CAD build for the part. Positions are in the model's coordinates, mm. A direction names the side the tool comes from. Coordinates: 2 decimals unless noted, no trailing zeros. Write each loop counter-clockwise with the first axis right and the second up, starting at its lowest first coordinate (ties: lowest second). Pieces come first, ordered by that corner, then holes. Notation, with made-up numbers: (15.5, 46) - (57.5, 46) arc R30 cw to (57.5, 80) - close; hole circle Ø8 at (10.5, 72). An arc over 180 degrees is marked (long way). One line per question, with ' | ' between items. Start each with the question number.
1. Which spindle directions (+Z, -Z, +X, -X, +Y, -Y) get a long thin tool onto all of the face, cutting with end or side? Do faces 1 (the cylindrical face through (66.182, 20.26, 100.327)), 2 (the flat face through (114.63, 10.353, 118.958)), 3 (the flat face through (103, 11, 0)). Say none if no direction does.
2. Band-saw the part on A-A, the plane x = 97. Write the cut outline in (y, z), then the cut area to 3 significant figures.
3. Two-plate mould, pull along X, no slides. Class faces 4 (the flat face through (0, 11, 92)), 5 (the cylindrical face through (66.182, 20.26, 170.327)), 6 (the flat face through (209, 10, 92)), 7 (the flat face through (103, 11, 187)): +X half, -X half, draft (parallel to the pull), parting line (faces both ways), or undercut.
4. Flat gauge pin, fed straight in: P1, Ø3.5, axis at x = 164, z = 102, coming from the +Y side. Where does the tip first touch, or does it go through?
5. Probe line 1 (Z direction, x = 164, y = 20.3); line 2 (X direction, y = 20, z = 172); line 3 (X direction, y = 15, z = 139). List the from-to ranges inside material, lowest first.
Autodesk Fusion 360 part; units mm, degrees
sketch "Smartie Feed" plane through (0, 0, 0) normal (0, 0, 1) x (1, 0, 0)
  line L0 (0, 0) -> (209, 0)
  line L1 (209, 0) -> (209, 21)
  line L2 (209, 21) -> (0, 21)
  line L3 (0, 21) -> (0, 0)
  dimension "d1" = 209
  dimension "d2" = 21
extrude "Extrude1" add sketch "Smartie Feed" along normal blind 187
sketch "Outlet" plane through (0, 0, 0) normal (0, -1, 0) x (1, 0, 0)
  line L0 (0, 0) -> (209, 0)
  line L1 (209, 0) -> (209, 187)
  line L2 (209, 187) -> (0, 187)
  line L3 (0, 187) -> (0, 0)
  line L4 (69, 146) -> (159, 146)
  line L5 (159, 146) -> (159, 116)
  line L6 (159, 116) -> (69, 116)
  line L7 (69, 116) -> (69, 146)
  dimension "d31" = 30
  dimension "d32" = 90
  dimension "d33" = 69
  dimension "d34" = 50
  dimension "d35" = 41
sketch "Inlet" plane through (0, 21, 0) normal (0, 1, 0) x (-1, 0, 0)
  line L0 (-209, 0) -> (0, 0)
  line L1 (0, 0) -> (0, 187)
  line L2 (0, 187) -> (-209, 187)
  line L3 (-209, 187) -> (-209, 0)
  line L4 (-69, 152) -> (-159, 152)
  line L5 (-159, 152) -> (-159, 122)
  line L6 (-159, 122) -> (-69, 122)
  line L7 (-69, 122) -> (-69, 152)
  dimension "d36" = 90
  dimension "d37" = 69
  dimension "d38" = 30
  dimension "d39" = 35
  dimension "d40" = 50
loft "Loft9" cut profiles "Inlet", "Outlet" section 1 contours L4 L5 L6 L7 section 2 contours L4 L5 L6 L7
sketch "Sketch6" plane through (0, 21, 0) normal (0, 1, 0) x (-1, 0, 0)
  line L0 (-69, 152) -> (-69, 122)
  line L1 (-69, 122) -> (-159, 122)
  line L2 (-159, 122) -> (-159, 152)
  line L3 (-159, 152) -> (-69, 152)
  line L4 (-209, 0) -> (0, 0)
  line L5 (0, 0) -> (0, 187)
  line L6 (0, 187) -> (-209, 187)
  line L7 (-209, 187) -> (-209, 0)
  circle A0 centre (-164, 172) radius 2.75
  circle A1 centre (-64, 172) radius 2.75
  circle A2 centre (-164, 102) radius 2.75
  circle A3 centre (-64, 102) radius 2.75
  dimension "d43" = 5.5
  dimension "d44" = 5.5
  dimension "d45" = 5.5
  dimension "d46" = 5.5
  dimension "d49" = 64
  dimension "d50" = 64
  dimension "d51" = 164
  dimension "d52" = 164
  dimension "d53" = 20
  dimension "d54" = 20
  dimension "d55" = 20
  dimension "d56" = 20
extrude "Extrude2" cut sketch "Sketch6" against normal blind 1.5 contours A0 | A1 | A2 | A3
equation "d1 = 219 mm - 10 mm"
equation "d3 = 166 mm + 21 mm"
equation "outletHeight = 15 mm"
equation "outletWidth = 20 mm"
equation "sortedContainersMidpointWidth = sortedContainersWidth + polycarbonateThickness"
equation "sortedContainersWidth = 60 mm"
equation "sortedContainersHeight = 113 mm"
equation "polycarbonateThickness = 6 mm"
equation "sortedContainersMidpointHeight = sortedContainersHeight + polycarbonateThickness"
equation "d33 = 90 mm - 21 mm"
equation "d35 = 30 mm - 21 mm + 5 mm + 6 mm + 21 mm"
equation "d37 = 90 mm - 21 mm"
equation "d39 = 30 mm - 21 mm + 5 mm + 21 mm"
equation "magnetDiameter = 5 mm"
equation "magnetHeight = 1.5 mm"
equation "d43 = magnetDiameter + 0.5 mm"
equation "d44 = magnetDiameter + 0.5 mm"
equation "d45 = magnetDiameter + 0.5 mm"
equation "d46 = magnetDiameter + 0.5 mm"
equation "d49 = 75 mm - 21 mm + 10 mm"
equation "d50 = 75 mm - 21 mm + 10 mm"
equation "d51 = 195 mm - 10 mm - 21 mm"
equation "d52 = 195 mm - 10 mm - 21 mm"
Filled in:
1) face 1: +Y | face 2: -Y | face 3: -Z, +X, -X, +Y, -Y
2) outline: (0, 0) - (21, 0) - (21, 122) - (0, 116) - close; (0, 146) - (21, 152) - (21, 187) - (0, 187) - close | area: 3,300 mm²
3) face 4: -X half | face 5: undercut | face 6: +X half | face 7: draft
4) P1: stops at y = 19.5
5) line 1: z = 0 to 99.25, 104.75 to 169.25, 174.75 to 187 | line 2: x = 0 to 61.25, 66.75 to 161.25, 166.75 to 209 | line 3: x = 0 to 69, 159 to 209
